The model under review builds one solid part; all positions refer to its coordinate system, in mm. Face numbers are marked on the shaded views. Round coordinates to 2 decimals unless told otherwise and drop trailing zeros. Order: outer loops, then holes, each group sorted by start corner. A loop starts at its lowest first (then second) coordinate and runs counter-clockwise, first axis right, second up.
1) Consider section D-D (x = -37.5). Give the boundary of the cut face in (y, z).
2) To check wall thickness, follow L1, parallel to Y at x = 23, z = 2.75; L2, parallel to Y at x = 0, z = 8; L3, parallel to X at y = 32.5, z = 2.75. State the ranges of each line that lie inside material, in increasing order.
3) Clearance check with flat-ended pins moving along their axes: P1, Ø1, axis at x = 21.5, z = 1.5, coming from the +Y side; P2, Ø2, axis at y = -19.5, z = 2, coming from the -X side; P3, Ø3, axis at x = -6.5, z = 8.5, coming from the -Y side. State where each tip first meets the part, or that it passes through.
4) Consider section C-C (y = 25). Give the boundary of the cut face in (x, z).
5) Consider section B-B (z = 6.5). Give the number of separate pieces and of enclosed holes in the cut face, then the cut area to 3 significant figures.
6) Mouldability with a two-part tool opening along X and no side actions: class the marked faces 1 and 2 as pulls with the +X half, pulls with the -X half, needs draft (parallel to the pull), parting line crosses it, or undercut.
7) Consider section A-A (x = 0). Give the boundary of the cut face in (y, z), then the cut area to 3 significant figures.
from build123d import *

# Parameters (mm, degrees)
SKETCH_1_R          = 50
EXTRUDE_1_DEPTH     = 10
SKETCH_4_R          = 8
CUT_EXTRUDE_3_DEPTH = 10
SKETCH_5_R          = 2
CUT_EXTRUDE_4_DEPTH = 10
SKETCH_6_R          = 3.38
CUT_EXTRUDE_5_DEPTH = 72.414284285


with BuildPart() as part:
    # 스케치1 → 보스-돌출1 (new body)
    with BuildSketch(Plane.XY):
        Circle(SKETCH_1_R)
    extrude(amount=EXTRUDE_1_DEPTH)

    # 스케치4 → 컷-돌출3 (cut)
    with BuildSketch(Plane.XY.offset(10)):
        Circle(SKETCH_4_R)
    extrude(amount=-CUT_EXTRUDE_3_DEPTH, mode=Mode.SUBTRACT)

    # 스케치5 → 컷-돌출4 (cut)
    with BuildSketch(Plane.XY.offset(10)):
        with Locations((-23, 8)):
            Circle(SKETCH_5_R)
        with Locations(Location((23, 8, 0), (0, 0, 180))):
            Circle(SKETCH_5_R)
        with Locations((23, -8)):
            Circle(SKETCH_5_R)
        with Locations(Location((-23, -8, 0), (0, 0, 180))):
            Circle(SKETCH_5_R)
    extrude(amount=-CUT_EXTRUDE_4_DEPTH, mode=Mode.SUBTRACT)

    # 스케치6 → 컷-돌출5 (cut, through all)
    with BuildSketch(Plane.XY.offset(10)):
        with Locations((0, 50)):
            Circle(SKETCH_6_R)
        with Locations((8.682408883, 49.240387651)):
            Circle(SKETCH_6_R)
        with Locations((17.101007166, 46.984631039)):
            Circle(SKETCH_6_R)
        with Locations((25, 43.301270189)):
            Circle(SKETCH_6_R)
        with Locations((32.139380484, 38.302222156)):
            Circle(SKETCH_6_R)
        with Locations((38.302222156, 32.139380484)):
            Circle(SKETCH_6_R)
        with Locations((43.301270189, 25)):
            Circle(SKETCH_6_R)
        with Locations((46.984631039, 17.101007166)):
            Circle(SKETCH_6_R)
        with Locations((49.240387651, 8.682408883)):
            Circle(SKETCH_6_R)
        with Locations((50, 0)):
            Circle(SKETCH_6_R)
        with Locations((49.240387651, -8.682408883)):
            Circle(SKETCH_6_R)
        with Locations((46.984631039, -17.101007166)):
            Circle(SKETCH_6_R)
        with Locations((43.301270189, -25)):
            Circle(SKETCH_6_R)
        with Locations((38.302222156, -32.139380484)):
            Circle(SKETCH_6_R)
        with Locations((32.139380484, -38.302222156)):
            Circle(SKETCH_6_R)
        with Locations((25, -43.301270189)):
            Circle(SKETCH_6_R)
        with Locations((17.101007166, -46.984631039)):
            Circle(SKETCH_6_R)
        with Locations((8.682408883, -49.240387651)):
            Circle(SKETCH_6_R)
        with Locations((0, -50)):
            Circle(SKETCH_6_R)
        with Locations((-8.682408883, -49.240387651)):
            Circle(SKETCH_6_R)
        with Locations((-17.101007166, -46.984631039)):
            Circle(SKETCH_6_R)
        with Locations((-25, -43.301270189)):
            Circle(SKETCH_6_R)
        with Locations((-32.139380484, -38.302222156)):
            Circle(SKETCH_6_R)
        with Locations((-38.302222156, -32.139380484)):
            Circle(SKETCH_6_R)
        with Locations((-43.301270189, -25)):
            Circle(SKETCH_6_R)
        with Locations((-46.984631039, -17.101007166)):
            Circle(SKETCH_6_R)
        with Locations((-49.240387651, -8.682408883)):
            Circle(SKETCH_6_R)
        with Locations((-50, 0)):
            Circle(SKETCH_6_R)
        with Locations((-49.240387651, 8.682408883)):
            Circle(SKETCH_6_R)
        with Locations((-46.984631039, 17.101007166)):
            Circle(SKETCH_6_R)
        with Locations((-43.301270189, 25)):
            Circle(SKETCH_6_R)
        with Locations((-38.302222156, 32.139380484)):
            Circle(SKETCH_6_R)
        with Locations((-32.139380484, 38.302222156)):
            Circle(SKETCH_6_R)
        with Locations((-25, 43.301270189)):
            Circle(SKETCH_6_R)
        with Locations((-17.101007166, 46.984631039)):
            Circle(SKETCH_6_R)
        with Locations((-8.682408883, 49.240387651)):
            Circle(SKETCH_6_R)
    extrude(amount=-CUT_EXTRUDE_5_DEPTH, mode=Mode.SUBTRACT)


solid = part.part
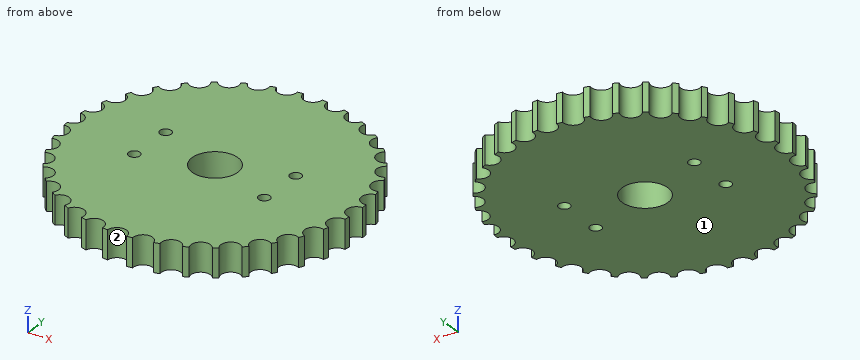
Answer below:
1. outline: (-28.86, 0) - (28.86, 0) - (28.86, 10) - (-28.86, 10) - close
2. L1: y = -40.58 to -10, -6 to 6, 10 to 40.58
2. L2: y = -46.62 to -8, 8 to 46.62
2. L3: x = -34.94 to 34.94
3. P1: stops at y = 45.38
3. P2: stops at x = -45.72
3. P3: stops at y = -49.75
4. outline: (-39.92, 0) - (39.92, 0) - (39.92, 10) - (-39.92, 10) - close
5. separate pieces: 1
5. enclosed holes: 5
5. area: 6,970 mm2
6. face 1: needs draft
6. face 2: undercut
7. outline: (-46.62, 0) - (-8, 0) - (-8, 10) - (-46.62, 10) - close; (8, 0) - (46.62, 0) - (46.62, 10) - (8, 10) - close
7. area: 772 mm2
